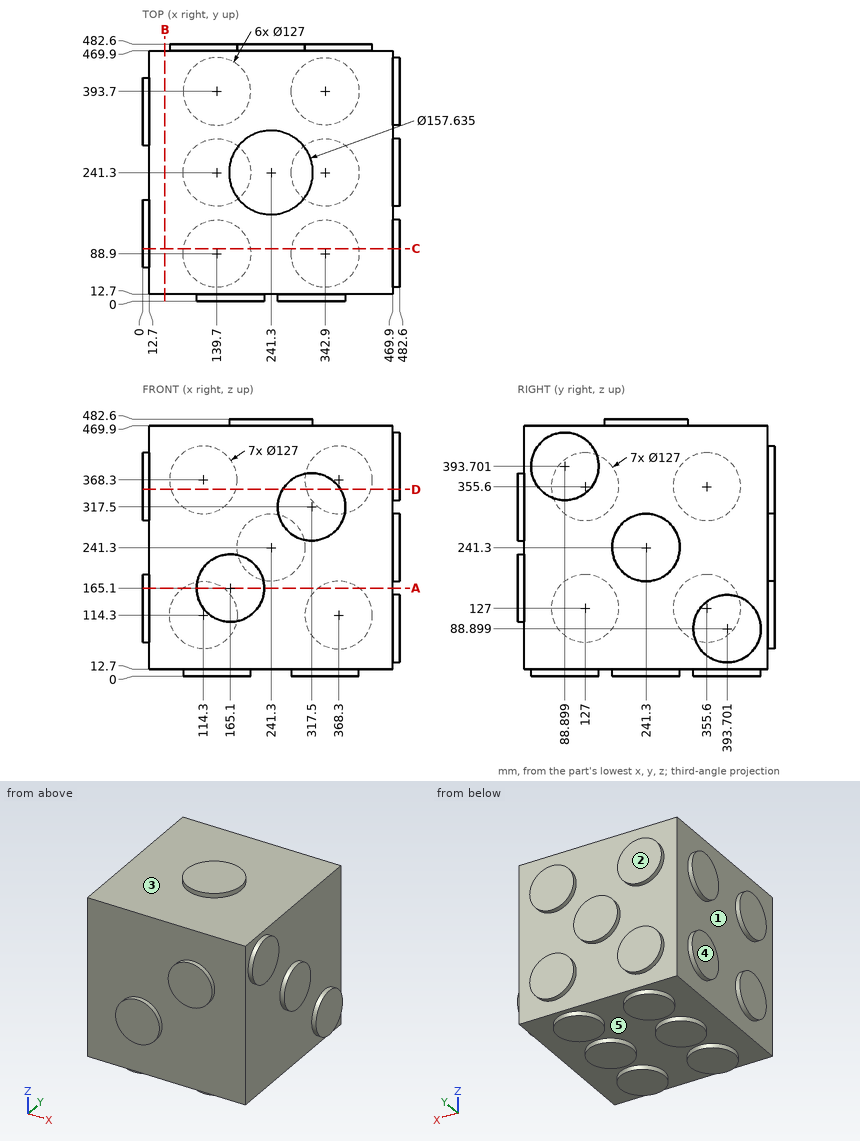
Job drawing, mm, ordinate dimensions from the low corner. One solid piece. A direction names the side the tool comes from. Coordinates: 2 decimals unless noted, no trailing zeros. Order: outer loops, then holes, each group sorted by start corner. A loop starts at its lowest first (then second) coordinate and runs counter-clockwise, first axis right, second up. Notation, with made-up numbers: (-23.5, 82) - (-10.5, 82) arc R22 ccw to (-10.5, 115) - close; hole circle Ø6 at (-6.5, 84). An arc over 180 degrees is marked (long way). Return JSON: item names as keys, results as strings. Group by question number.
1) Probe line 1 (Z direction, x = 367.5, y = 123); line 2 (Z direction, x = 45, y = 371). List the from-to ranges inside material, lowest first. Write a range as from..to.
2) Tool access for the marked faces 4 and 5: list every direction of +Z, -Z, +X, -X, +Y, -Y with a clear straight run to the whole face (end or side of a thin tool).
3) Flat gauge pins, fed straight in: P1, Ø10, axis at x = 281.5, z = 53, coming from the +Y side; P2, Ø2, axis at y = 173.5, z = 72, coming from the +X side; P3, Ø8, axis at x = 402, z = 254.5, coming from the -Y side. Where does each tip first touch, or does it go through?
4) Saw through at A-A, the plane z = 165.1. Write the cut outline in (x, y).
5) Saw through at D-D, the plane z = 350.5. Write the cut outline in (x, y) (1 decimal).
6) Mould opens along Z. For the marked faces 1, 2 and 3 say: released by +Z, released by -Z, zero draft, split by the parting line, or undercut.
7) Saw through at B-B, the plane x = 42. Write the cut outline in (y, z), plus the area to 3 significant figures.
8) Saw through at C-C, the plane y = 98.5. Write the cut outline in (x, z) (1 decimal), plus the area to 3 significant figures.
Values found:
{
 "1": {"line 1": "z = 0..469.9", "line 2": "z = 12.7..469.9"},
 "2": {"face 4": "+Z, -Z, -X, +Y, -Y", "face 5": "-Z"},
 "3": {"P1": "stops at y = 469.9", "P2": "stops at x = 469.9", "P3": "stops at y = 12.7"},
 "4": {"outline": "(0, 76.2) - (12.7, 76.2) - (12.7, 12.7) - (101.6, 12.7) - (101.6, 0) - (228.6, 0) - (228.6, 12.7) - (469.9, 12.7) - (469.9, 469.9) - (406.4, 469.9) - (406.4, 482.6) - (330.2, 482.6) - (330.2, 469.9) - (152.4, 469.9) - (152.4, 482.6) - (76.2, 482.6) - (76.2, 469.9) - (12.7, 469.9) - (12.7, 406.4) - (0, 406.4) - (0, 304.8) - (12.7, 304.8) - (12.7, 177.8) - (0, 177.8) - close"},
 "5": {"outline": "(0, 63.7) - (12.7, 63.7) - (12.7, 12.7) - (263.2, 12.7) - (263.2, 0) - (371.8, 0) - (371.8, 12.7) - (469.9, 12.7) - (469.9, 42.4) - (482.6, 42.4) - (482.6, 135.4) - (469.9, 135.4) - (469.9, 469.9) - (429.3, 469.9) - (429.3, 482.6) - (307.3, 482.6) - (307.3, 469.9) - (175.3, 469.9) - (175.3, 482.6) - (53.3, 482.6) - (53.3, 469.9) - (12.7, 469.9) - (12.7, 418.9) - (0, 418.9) - (0, 292.3) - (12.7, 292.3) - (12.7, 190.3) - (0, 190.3) - close"},
 "6": {"face 1": "undercut", "face 2": "zero draft", "face 3": "released by +Z"},
 "7": {"outline": "(12.7, 12.7) - (469.9, 12.7) - (469.9, 469.9) - (12.7, 469.9) - close", "area": "209,000 mm²"},
 "8": {"outline": "(0, 70.3) - (12.7, 70.3) - (12.7, 12.7) - (76.9, 12.7) - (76.9, 0) - (202.5, 0) - (202.5, 12.7) - (280.1, 12.7) - (280.1, 0) - (405.7, 0) - (405.7, 12.7) - (469.9, 12.7) - (469.9, 330.9) - (482.6, 330.9) - (482.6, 456.5) - (469.9, 456.5) - (469.9, 469.9) - (12.7, 469.9) - (12.7, 412.3) - (0, 412.3) - (0, 298.9) - (12.7, 298.9) - (12.7, 183.7) - (0, 183.7) - close", "area": "217,000 mm²"}
}
